from build123d import *

# Parameters (mm, degrees)
SKETCH_1_W          = 120
SKETCH_1_H          = 100
EXTRUDE_1_DEPTH     = 4
FILLET_1_R          = 14
SKETCH_7_R          = 2.5
CUT_EXTRUDE_2_DEPTH = 5
SKETCH_14_R         = 2
CUT_EXTRUDE_3_DEPTH = 5


with BuildPart() as part:
    # 草图1 → 凸台-拉伸1 (new body)
    with BuildSketch(Plane.XY):
        with Locations((7.34439834, -11.161825726)):
            Rectangle(SKETCH_1_W, SKETCH_1_H)
    extrude(amount=EXTRUDE_1_DEPTH)

    # 圆角1
    fillet_1_edges = [part.edges().sort_by_distance(p)[0] for p in [
        (-52.65560166, 38.838174274, 2),
        (67.34439834, 38.838174274, 2),
        (67.34439834, -61.161825726, 2),
        (-52.65560166, -61.161825726, 2),
    ]]
    fillet(fillet_1_edges, radius=FILLET_1_R)

    # 草图7 → 切除-拉伸2 (cut, through all)
    with BuildSketch(Plane(origin=(0, 0, 0), x_dir=(-1, 0, 0), z_dir=(0, 0, -1))):
        with Locations((15.15560166, -11.161825726)):
            Circle(SKETCH_7_R)
        with Locations((30.15560166, -11.161825726)):
            Circle(SKETCH_7_R)
    extrude(amount=-CUT_EXTRUDE_2_DEPTH, mode=Mode.SUBTRACT)

    # 草图14 → 切除-拉伸3 (cut, through all)
    with BuildSketch(Plane(origin=(0, 0, 0), x_dir=(-1, 0, 0), z_dir=(0, 0, -1))):
        with Locations((42.240931861, -49.965268324)):
            Circle(SKETCH_14_R)
        with Locations((20.240931861, -49.965268324)):
            Circle(SKETCH_14_R)
        with Locations((42.240931861, -36.965268324)):
            Circle(SKETCH_14_R)
        with Locations((20.240931861, -36.965268324)):
            Circle(SKETCH_14_R)
        with Locations((42.240931861, 14.942073)):
            Circle(SKETCH_14_R)
        with Locations((42.240931861, 27.942073)):
            Circle(SKETCH_14_R)
        with Locations((20.240931861, 14.942073)):
            Circle(SKETCH_14_R)
        with Locations((20.240931861, 27.942073)):
            Circle(SKETCH_14_R)
        with Locations((-14.259068139, -11.161825726)):
            Circle(SKETCH_14_R)
        with Locations((-37.759068139, -17.661825726)):
            Circle(SKETCH_14_R)
        with Locations((-59.759068139, -17.661825726)):
            Circle(SKETCH_14_R)
        with Locations((-59.759068139, -4.661825726)):
            Circle(SKETCH_14_R)
        with Locations((-37.759068139, -4.661825726)):
            Circle(SKETCH_14_R)
        with BuildLine():
            ThreePointArc((-1.760462288, -11.236489328), (-3.684404538, -9.163219875), (-5.75767399, -11.087162125))
            ThreePointArc((-5.75767399, -11.087162125), (-7.203940461, -16.202085414), (-10.83494306, -20.084088387))
            ThreePointArc((-10.83494306, -20.084088387), (-11.410230768, -22.85339228), (-8.640926875, -23.428679989))
            ThreePointArc((-8.640926875, -23.428679989), (-3.720371267, -18.167981055), (-1.760462288, -11.236489328))
        make_face()
    extrude(amount=-CUT_EXTRUDE_3_DEPTH, mode=Mode.SUBTRACT)


solid = part.part
Could you check a few things on this model? Use its own coordinates, in mm. A direction names the side the tool comes from. Round coordinates to 2 decimals unless told otherwise and drop trailing zeros. Write item = value, one per line.
1) If we mould it in two halves opening along Y, with no side actions, what happens to faces 1 (the flat face through (7, -61.162, 2)), 2 (the flat face through (-52.656, -12, 2)), 3 (the cylindrical face through (-32.54, -10.41, 1.97))? For each: pulls with the +Y half, pulls with the -Y half, needs draft (parallel to the pull), parting line crosses it, or undercut.
Computed:
face_1 = pulls with the -Y half
face_2 = needs draft
face_3 = undercut
2) Imagine slicing it at A-A (z = 1.9). Give the number of separate pieces and of enclosed holes in the cut face, and give its area (3 significant figures).
Computed:
separate_pieces = 1
enclosed_holes = 16
area = 11,600 mm2
3) I need wall thicknesses on line 1 along X through (y, z) = (-4.5, 0.6); line 2 along Y through (x, z) = (-22, 3.65); line 3 along X through (y, z) = (-47.5, 3.6). Which ranges of each line are inside material? Lowest first, please. Write a range as from..to.
Computed:
line_1 = -52.66..35.77, 39.75..57.77, 61.75..67.34
line_2 = -61.16..-50.92, -49.01..-37.92, -36.01..13.99, 15.89..26.99, 28.89..38.84
line_3 = -52.65..67.34
4) On a 3-axis mill with a long thin cutter (end or side, diameter ignored), from which of +Z, -Z, +X, -X, +Y, -Y can I reach the whole of each face in a straight line? I mean faces 4 (the cylindrical face through (7.17, -16.14, 1.97)), 5 (the flat face through (7, -10, 0)). Say none if no direction works.
Computed:
face_4 = +Z, -Z
face_5 = -Z, +X, -X, +Y, -Y
